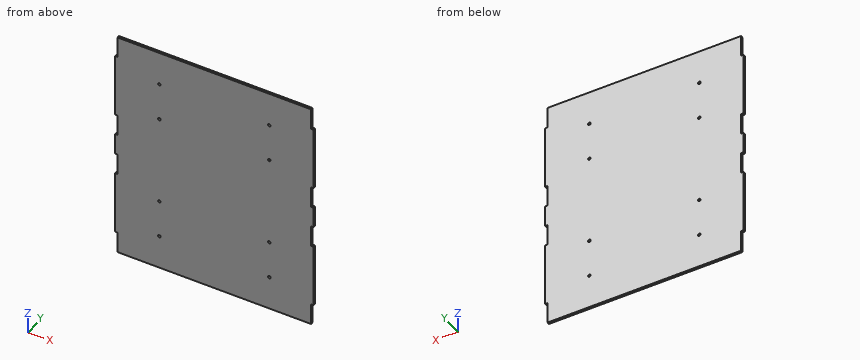
from build123d import *

# Parameters (mm, degrees)
CROQUIS1_R              = 1.7
SALIENTE_EXTRUIR1_DEPTH = 3


with BuildPart() as part:
    # Croquis1 → Saliente-Extruir1 (new body)
    with BuildSketch(Plane(origin=(0, 0, 0), x_dir=(1, 0, 0), z_dir=(0, 1, 0))):
        Polygon((-97.174990899, 154.00569786), (152.825009101, 154.00569786), (152.825009101, 126.00569786), (155.825009101, 126.00569786), (155.825009101, 42.00569786), (152.825009101, 42.00569786), (152.825009101, 14.00569786), (155.825009101, 14.00569786), (155.825009101, -13.99430214), (152.825009101, -13.99430214), (152.825009101, -41.99430214), (155.825009101, -41.99430214), (155.825009101, -125.99430214), (152.825009101, -125.99430214), (152.825009101, -153.99430214), (-97.174990899, -153.99430214), (-97.174990899, -125.99430214), (-100.174990899, -125.99430214), (-100.174990899, -41.99430214), (-97.174990899, -41.99430214), (-97.174990899, -13.99430214), (-100.174990899, -13.99430214), (-100.174990899, 14.00569786), (-97.174990899, 14.00569786), (-97.174990899, 42.00569786), (-100.174990899, 42.00569786), (-100.174990899, 126.00569786), (-97.174990899, 126.00569786), align=None)
        with Locations((-43.174990899, 109.01139572)):
            Circle(CROQUIS1_R, mode=Mode.SUBTRACT)
        with Locations((-43.174990899, 59)):
            Circle(CROQUIS1_R, mode=Mode.SUBTRACT)
        with Locations((-43.174990899, -58.99430214)):
            Circle(CROQUIS1_R, mode=Mode.SUBTRACT)
        with Locations((-43.174990899, -108.99430214)):
            Circle(CROQUIS1_R, mode=Mode.SUBTRACT)
        with Locations((98.825009101, 59)):
            Circle(CROQUIS1_R, mode=Mode.SUBTRACT)
        with Locations((98.825009101, 109.01139572)):
            Circle(CROQUIS1_R, mode=Mode.SUBTRACT)
        with Locations((98.825009101, -108.99430214)):
            Circle(CROQUIS1_R, mode=Mode.SUBTRACT)
        with Locations((98.825009101, -58.99430214)):
            Circle(CROQUIS1_R, mode=Mode.SUBTRACT)
    extrude(amount=SALIENTE_EXTRUIR1_DEPTH)


solid = part.part
Verification items for the finished model (mm, model axes). Give positions to 0.01 mm unless a question says otherwise; leave off trailing zeros. Order: outer loops, then holes, each group sorted by start corner. A loop starts at its lowest first (then second) coordinate and runs counter-clockwise, first axis right, second up. Notation, with made-up numbers: (47.5, 65) -> (69.5, 65) arc R25 ccw to (69.5, 86) -> close; hole circle Ø9 at (38.25, -29). An arc over 180 degrees is marked (long way). Answer as CSV lines item,"result".
Q1. Sectioned sample at A-A on z = 28. Record the cut outline in (x, y) (3 decimals).
Solutions:
outline,"(-97.175, 0) -> (152.825, 0) -> (152.825, 3) -> (-97.175, 3) -> close"
Q2. Depth check by flat-ended pin: pin 1 (1 mm diameter, centred on x = -41.5, z = 5.5, fed in from -Y); pin 2 (1.5 mm diameter, centred on y = 2, z = -144, fed in from +X) (3 decimals); pin 3 (1.5 mm diameter, centred on y = 1.5, z = 27, fed in from -X) (3 decimals); pin 4 (1.5 mm diameter, centred on x = -98.5, y = 2, fed in from -Z). Enter the tip coordinate at first touch or a pass-through.
Solutions:
pin 1,"stops at y = 0"
pin 2,"stops at x = 152.825"
pin 3,"stops at x = -97.175"
pin 4,"stops at z = -126.01"
Q3. Scan lines: probe 1 along X at (y, z) = (0.4, -108.5) (3 decimals); probe 2 along X at (y, z) = (2.1, -59) (3 decimals); probe 3 along X at (y, z) = (1.9, 126.5) (3 decimals). Record each from-to range of solid material in increasing order.
Solutions:
probe 1,"x = -100.175 to -44.796, -41.554 to 97.204, 100.446 to 155.825"
probe 2,"x = -100.175 to -44.875, -41.475 to 97.125, 100.525 to 155.825"
probe 3,"x = -97.175 to 152.825"
